Could you check a few things on this drawing? It's one solid part, dimensions in mm from its lowest x, y, z. A direction names the side the tool comes from. Give positions to 0.01 mm unless a question says otherwise; leave off trailing zeros. Order: outer loops, then holes, each group sorted by start corner. A loop starts at its lowest first (then second) coordinate and runs counter-clockwise, first axis right, second up. Notation, with made-up numbers: M 77,49.25 L 88,49.25 A23 ccw 88,71.25 Z; hole C -7,-31.75 d5. An arc over 180 degrees is marked long. Use one line per item in the form item = value. Start each with the question number.
1. Will these pins go through, and if not, where does the flat tip stop? P1, Ø3.5, axis at x = 18, z = 5, coming from the -Y side; P2, Ø4.5, axis at x = 39, z = 2, coming from the +Y side; P3, Ø3, axis at x = 6, z = 5, coming from the +Y side.
2. For the marked faces 1, 2 and 3, which set-ups out of +Z, -Z, +X, -X, +Y, -Y let a thin tool reach every point of the face, with its end or its side?
3. I want a section at C-C, the plane y = 3.75. List the corners of the cut face in (x, z) for me, and give its area (3 significant figures).
4. I want a section at A-A, the plane x = 4.5. List the corners of the cut face in (y, z) for me.
5. I want a section at D-D, the plane y = 6.75. List the corners of the cut face in (x, z) for me, and give its area (3 significant figures).
6. I want a section at B-B, the plane z = 1.25. Count the separate pieces of the cut face and the enclosed holes in it, and give its area (3 significant figures).
7. I need wall thicknesses on L1, parallel to X at y = 3.25, z = 1.75; L2, parallel to X at y = 8.25, z = 2.5. Which ranges of each line are inside material? Lowest first, please.
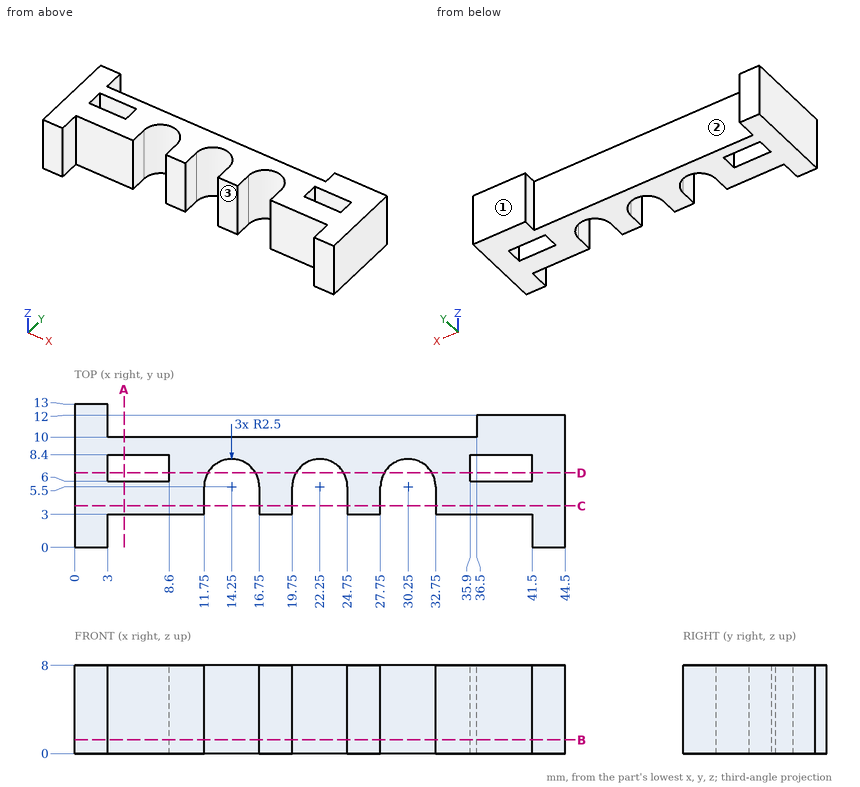
Check result:
q1.P1 = 3
q1.P2 = 12
q1.P3 = 10
q2.face_1 = +Z, -Z, +X, +Y
q2.face_2 = +Z, -Z, +Y
q2.face_3 = +Z, -Z, -Y
q3.outline = M 0,0 L 11.75,0 L 11.75,8 L 0,8 Z; M 16.75,0 L 19.75,0 L 19.75,8 L 16.75,8 Z; M 24.75,0 L 27.75,0 L 27.75,8 L 24.75,8 Z; M 32.75,0 L 44.5,0 L 44.5,8 L 32.75,8 Z
q3.area = 236 mm2
q4.outline = M 3,0 L 6,0 L 6,8 L 3,8 Z; M 8.4,0 L 10,0 L 10,8 L 8.4,8 Z
q5.outline = M 0,0 L 3,0 L 3,8 L 0,8 Z; M 8.6,0 L 12.08,0 L 12.08,8 L 8.6,8 Z; M 16.42,0 L 20.08,0 L 20.08,8 L 16.42,8 Z; M 24.42,0 L 28.08,0 L 28.08,8 L 24.42,8 Z; M 32.42,0 L 35.9,0 L 35.9,8 L 32.42,8 Z; M 41.5,0 L 44.5,0 L 44.5,8 L 41.5,8 Z
q5.area = 162 mm2
q6.separate_pieces = 1
q6.enclosed_holes = 2
q6.area = 261 mm2
q7.L1 = 0 to 11.75, 16.75 to 19.75, 24.75 to 27.75, 32.75 to 44.5
q7.L2 = 0 to 3, 8.6 to 35.9, 41.5 to 44.5
